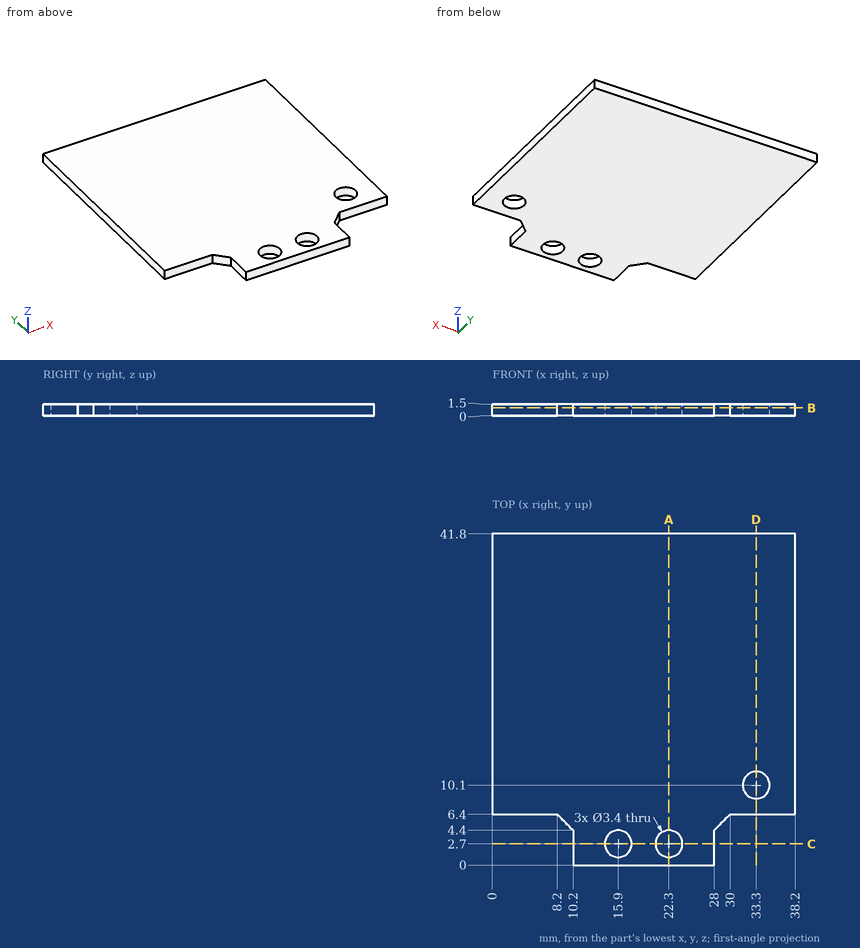
Print and shaded views of the part. All mm, measured from the part's lowest x, y and z. Give positions to 0.01 mm unless a question says otherwise; leave off trailing zeros. Loops run counter-clockwise (first coordinate to the right, second up) from the corner with the lowest first, then second, coordinate; pieces in that order, holes last. Notation, with made-up numbers: M 4.5,-10 L 32.5,-10 A25 cw 32.5,24 Z; hole C 84.5,23.25 d7. An arc over 180 degrees is marked long. Write each question's results on one line, items separated by ' | '.
Q1. Band-saw the part on D-D on x = 33.3. Write the cut outline in (y, z).
Geometry check:
outline: M 6.4,0 L 8.4,0 L 8.4,1.5 L 6.4,1.5 Z; M 11.8,0 L 41.8,0 L 41.8,1.5 L 11.8,1.5 Z
Q2. Probe probe 1 along Y at (x, z) = (22.3, 1.25); probe 2 along Y at (x, z) = (33.3, 0.7); probe 3 along Y at (x, z) = (4, 0.2). List the from-to ranges inside material, lowest first.
Geometry check:
probe 1: y = 0 to 1, 4.4 to 41.8 | probe 2: y = 6.4 to 8.4, 11.8 to 41.8 | probe 3: y = 6.4 to 41.8
Q3. Band-saw the part on C-C on y = 2.7. Write the cut outline in (x, z), and give its area (3 significant figures).
Geometry check:
outline: M 10.2,0 L 14.2,0 L 14.2,1.5 L 10.2,1.5 Z; M 17.6,0 L 20.6,0 L 20.6,1.5 L 17.6,1.5 Z; M 24,0 L 28,0 L 28,1.5 L 24,1.5 Z | area: 16.5 mm²
Q4. Band-saw the part on A-A on x = 22.3. Write the cut outline in (y, z).
Geometry check:
outline: M 0,0 L 1,0 L 1,1.5 L 0,1.5 Z; M 4.4,0 L 41.8,0 L 41.8,1.5 L 4.4,1.5 Z
Q5. Band-saw the part on B-B on z = 1. Write the cut outline in (x, y), and give its area (3 significant figures).
Geometry check:
outline: M 0,6.4 L 8.2,6.4 L 10.2,4.4 L 10.2,0 L 28,0 L 28,4.4 L 30,6.4 L 38.2,6.4 L 38.2,41.8 L 0,41.8 Z; hole C 15.9,2.7 d3.4; hole C 22.3,2.7 d3.4; hole C 33.3,10.1 d3.4 | area: 1,440 mm²
